Autodesk Inventor part; units mm, degrees
ref_plane "YZ Plane" through (0, 0, 0) normal (1, 0, 0) x (0, 1, 0)
ref_plane "XZ Plane" through (0, 0, 0) normal (0, 1, 0) x (-1, 0, 0)
ref_plane "XY Plane" through (0, 0, 0) normal (0, 0, 1) x (1, 0, 0)
sketch "Sketch1" plane through (0, 0, 0) normal (1, 0, 0) x (0, 1, 0)
  line L0 (-57.15, 14.351) -> (12.7, 14.351)
  line L1 (12.7, 14.351) -> (12.7, -14.351)
  line L2 (12.7, -14.351) -> (-12.7, -14.351)
  line L3 (-12.7, -14.351) -> (-12.7, -20.701)
  line L4 (-12.7, -20.701) -> (19.05, -20.701)
  line L5 (19.05, -20.701) -> (19.05, 19.431)
  line L6 (19.05, 19.431) -> (-23.8064, 19.431)
  arc A0 (-36.322, 50.927) -> (-36.322, 38.735) centre (-38.1, 44.831) ccw
  arc A1 (-36.322, 50.927) -> (-31.3296, 51.5467) centre (-34.544, 57.023) ccw
  arc A2 (-35.433, 53.975) -> (-47.5727, 43.8339) centre (-38.1, 44.831) ccw
  arc A3 (-57.15, 14.351) -> (-47.5727, 43.8339) centre (-85.4633, 39.8454) ccw
  arc A4 (-35.433, 53.975) -> (-32.9368, 54.2848) centre (-34.544, 57.023) ccw
  line L7 (-32.9368, 54.2848) -> (-31.3296, 51.5467)
  arc A5 (-31.3296, 38.1153) -> (-36.322, 38.735) centre (-34.544, 32.639) ccw
  line L8 (-31.3296, 38.1153) -> (-32.9368, 35.3772)
  line L9 (-38.1, 44.831) -> (-26.6352, 44.831) construction
  arc A6 (-32.9368, 35.3772) -> (-23.8064, 19.431) centre (-23.8064, 30.018) ccw
  point P0 (0, 0)
  point P1 (12.7, 0)
  dimension "d0" = 5.08
  dimension "d1" = 3.175
  dimension "d2" = 38.1
  dimension "d3" = 6.35
  dimension "d5" = 6.35
  dimension "d7" = 50.8
  dimension "d8" = 6.35
  dimension "d9" = 6.35
  dimension "d11" = 19.05
  dimension "d12" = 12.7
  dimension "d13" = 25.4
  dimension "d14" = 28.702
  dimension "d15" = 6.35
  dimension "d16" = 12.192
  dimension "d17" = 25.4
extrude "Extrusion1" add sketch "Sketch1" along normal blind 12.7
fillet "Fillet1" radius 9.525 4 edges at (6.35, 12.7, 14.351) (6.35, 12.7, -14.351) (6.35, 19.05, 19.431) (6.35, 19.05, -20.701)
fillet "Fillet2" radius 1.5875 3 edges at (6.35, -31.3296, 51.5467) (6.35, -32.9368, 54.2848) (6.35, -31.3296, 38.1153)
equation "\"d15\" = d3"
equation "\"d16\" = 1.92 * d5"
properties part number "Curtain Adapter"
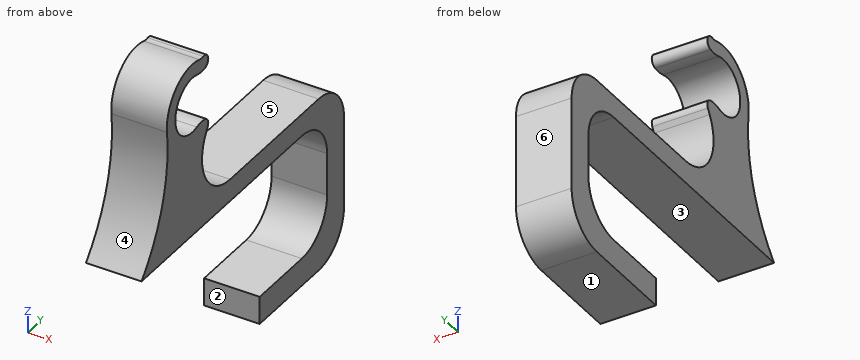
The listing builds one solid part. Answer for the finished solid, in the listing's coordinates (mm). Face numbers are marked on the shaded views. A direction names the side the tool comes from. Give positions to 0.01 mm unless a question says otherwise; leave off trailing zeros. Order: outer loops, then holes, each group sorted by start corner. A loop starts at its lowest first (then second) coordinate and runs counter-clockwise, first axis right, second up. Notation, with made-up numbers: M 67.25,27 L 89.25,27 A28 cw 89.25,46 Z; hole C 26,-38 d7. An arc over 180 degrees is marked long. Put each result on its own line as item: value. Start each with the question number.
Item 1: The part is cut by section A-A, the plane y = -38.1. Determine the outline of the cut face in (x, z).
Item 2: The part is cut by section C-C, the plane z = 37.5. Determine the outline of the cut face in (x, y).
Item 3: Which of the six approach directions +Z, -Z, +X, -X, +Y, -Y give full straight-line access (tool end or side, diameter ignored) to the marked faces 1, 2 and 3?
Item 4: Flat-ended cylindrical pins translate along their axes: P1, Ø2, axis at x = 10, z = -6.5, coming from the -Y side; P2, Ø3, axis at x = 9.5, z = -1.5, coming from the -Y side; P3, Ø4, axis at x = 4.5, y = -5.5, coming from the +Z side; P4, Ø2, axis at y = 11.5, z = 1.5, coming from the +X side. Find the tip coordinate at first contact, or state that the pin passes through.
Item 5: For a pull along Z with two mould halves and no side action, classify the marked faces 4, 5 and 6 as +Z half, -Z half, draft (parallel to the pull), parting line (faces both ways), or undercut.
Item 6: Find the intervals of material crossed by line 1 along Z through (x, y) = (7.75, -38.1); line 2 along Z through (x, y) = (8.75, -7); line 3 along Y through (x, z) = (11.5, -0.5), in increasing order.
Item 7: The part is cut by section D-D, the plane y = -22. Determine the outline of the cut face in (x, z), and give its area (3 significant figures).
Answer key:
1. outline: M 0,14.35 L 12.7,14.35 L 12.7,38.48 L 0,38.48 Z; M 0,51.18 L 12.7,51.18 L 12.7,54.36 L 0,54.36 Z
2. outline: M 0,-47.44 L 12.7,-47.44 L 12.7,-32.06 L 0,-32.06 Z
3. face 1: -Z, +X, -X, +Y, -Y
3. face 2: -Z, +X, -X, -Y
3. face 3: +X, -X, -Y
4. P1: stops at y = 12.32
4. P2: stops at y = 12.7
4. P3: stops at z = 19.43
4. P4: passes through
5. face 4: undercut
5. face 5: +Z half
5. face 6: draft
6. line 1: z = 14.35 to 38.48, 51.18 to 54.36
6. line 2: z = -20.7 to -14.35, 14.35 to 19.43
6. line 3: y = 12.7 to 19.05
7. outline: M 0,14.35 L 12.7,14.35 L 12.7,19.43 L 0,19.43 Z
7. area: 64.5 mm²
